The drawing under review shows one solid part. Ordinate dimensions are in mm from its lowest x, y, z. A direction names the side the tool comes from. Coordinates: 2 decimals unless noted, no trailing zeros. Order: outer loops, then holes, each group sorted by start corner. A loop starts at its lowest first (then second) coordinate and runs counter-clockwise, first axis right, second up. Notation, with made-up numbers: (-3, -4) - (16, -4) arc R24 ccw to (16, 19) - close; hole circle Ø10 at (29, 74). An arc over 180 degrees is marked (long way). Write each question's results on one line, items separated by ' | '. Start each with the question number.
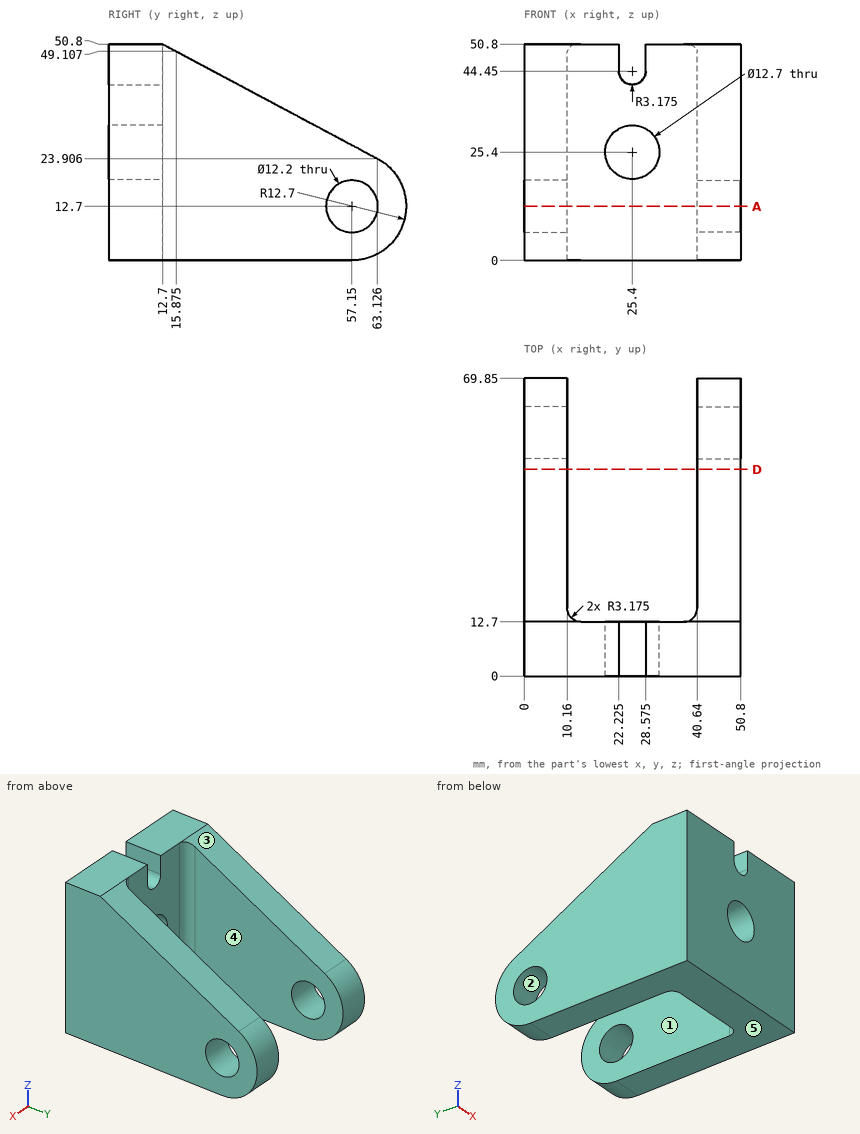
(1) Take a section at D-D (y = 48.5). State the section outline as (x, z) points.
(2) Clearance check with flat-ended pins moving along their axes: pin 1 (5 mm diameter, centred on x = 32, y = 16, fed in from -Z); pin 2 (7 mm diameter, centred on x = 21.5, z = 13, fed in from +Y). State where each tip first meets the part, or that it passes through.
(3) Tool access review of the marked faces 4 and 5: name each direction out of +Z, -Z, +X, -X, +Y, -Y from which nothing blocks a thin tool from reaching the whole face with its end or side.
(4) To check wall thickness, follow line 1 along X through (y, z) = (10.5, 47) (1 decimal); line 2 along X through (y, z) = (39, 16); line 3 along Y through (x, z) = (7, 12.7). State the ranges of each line that lie inside material, in increasing order. Write a range as [from, to].
(5) Mouldability with a two-part tool opening along Z and no side actions: class the marked faces 1, 2 and 3 as +Z half, -Z half, draft (parallel to the pull), parting line (faces both ways), or undercut.
(6) Take a section at A-A (z = 12.7). State how many separate pieces and enclosed holes the cut face has, plus the area to 3 significant figures.
Worked out:
1) outline: (0, 0) - (10.16, 0) - (10.16, 31.71) - (0, 31.71) - close; (40.64, 0) - (50.8, 0) - (50.8, 31.71) - (40.64, 31.71) - close
2) pin 1: through | pin 2: y = 12.7
3) face 4: +Z, -Z, +Y | face 5: -Z, +X, -X, +Y, -Y
4) line 1: [0, 22.2], [28.6, 50.8] | line 2: [0, 10.16], [40.64, 50.8] | line 3: [0, 51.05], [63.25, 69.85]
5) face 1: draft | face 2: undercut | face 3: +Z half
6) separate pieces: 3 | enclosed holes: 0 | area: 1,560 mm^2
